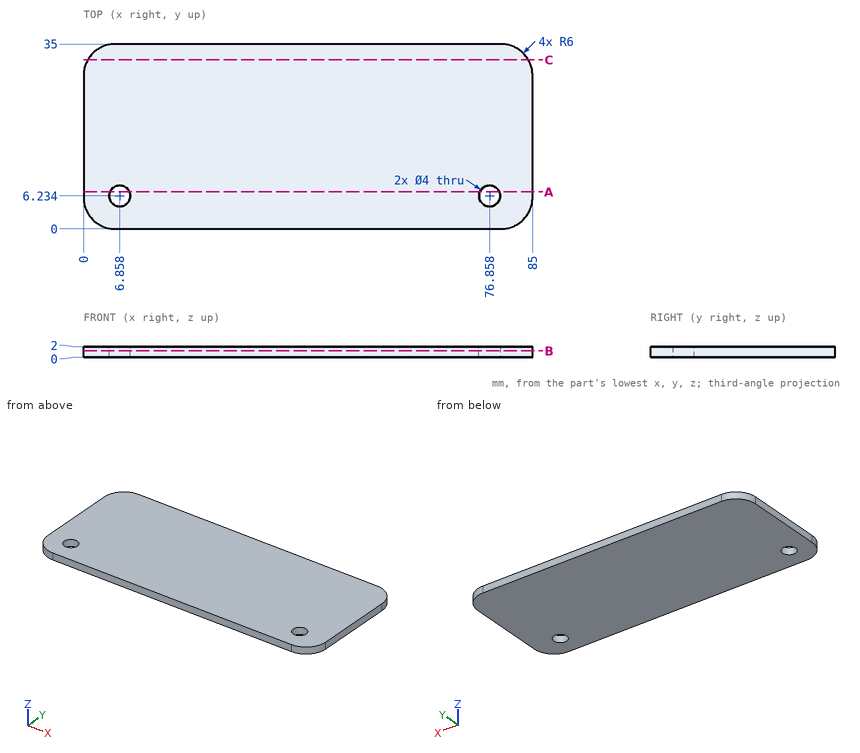
Check sheet for the drawn part. Datum: minimum x, y, z corner. Units: mm. Round coordinates to 2 decimals unless told otherwise and drop trailing zeros. Order: outer loops, then holes, each group sorted by start corner. A loop starts at its lowest first (then second) coordinate and runs counter-clockwise, first axis right, second up. Notation, with made-up numbers: M -25.5,65 L 9.5,65 A28 cw 9.5,84 Z; hole C -21.75,-21.75 d11. An arc over 180 degrees is marked long. Write each question's results on one line, items separated by ' | '. Start each with the question number.
1. Cross-section at B-B on z = 1.25. Record the boundary of the cut face in (x, y).
2. Material ranges on L1, parallel to Y at x = 5.5, z = 1.35 (1 decimal); L2, parallel to X at y = 29.5, z = 0.35; L3, parallel to X at y = 3.5, z = 0.9 (1 decimal), recorded low to high. Write a range as from..to.
3. Cross-section at C-C on y = 32. Record the boundary of the cut face in (x, z).
4. Cross-section at A-A on y = 7. Record the boundary of the cut face in (x, z) (1 decimal), plus the area to 3 significant figures.
5. Go/stop test with a flat-tipped pin: P1, Ø4.5, axis at x = 76.86, y = 6.23, coming from the +Z side. Record where the tip stops, or that it passes through.
Resolved:
1) outline: M 0,6 A6 ccw 6,0 L 79,0 A6 ccw 85,6 L 85,29 A6 ccw 79,35 L 6,35 A6 ccw 0,29 Z; hole C 6.86,6.23 d4; hole C 76.86,6.23 d4
2) L1: 0..4.8, 7.7..35 | L2: 0.02..84.98 | L3: 0.5..84.5
3) outline: M 0.8,0 L 84.2,0 L 84.2,2 L 0.8,2 Z
4) outline: M 0,0 L 5,0 L 5,2 L 0,2 Z; M 8.7,0 L 75,0 L 75,2 L 8.7,2 Z; M 78.7,0 L 85,0 L 85,2 L 78.7,2 Z | area: 155 mm2
5) P1: z = 2
